Build history of the part. All positions in model axes, mm. A direction names the side the tool comes from. Round coordinates to 2 decimals unless told otherwise and drop trailing zeros. Loops run counter-clockwise (first coordinate to the right, second up) from the corner with the lowest first, then second, coordinate; pieces in that order, holes last. Notation, with made-up numbers: (-38.5, -8) - (-24.5, -8) arc R21 ccw to (-24.5, 24) - close; hole circle Ø7 at (2.25, 89). An arc over 180 degrees is marked (long way). Put each result on its own line as item: value. Start each with the question number.
from build123d import *

# Parameters (mm, degrees)
SKETCH_1_R               = 16.3
EXTRUDE_1_DEPTH          = 19.75
SKETCH_2_W               = 36.5
SKETCH_2_H               = 2.5
EXTRUDE_2_DEPTH          = 39.5
SKETCH_3_W               = 44.844436064
SKETCH_3_H               = 25.506740045
CUT_EXTRUDE_1_DEPTH      = 50
EXTRUDE_3_DEPTH          = 5.05
SKETCH_5_R               = 14.25
CUT_EXTRUDE_2_DEPTH      = 29.4
SKETCH_6_R               = 2.5
CUT_EXTRUDE_3_DEPTH      = 44.930797853
CUT_EXTRUDE_6_REACH      = 49.993
SKETCH_9_R               = 7.5
SKETCH_12_R              = 1.15
CUT_EXTRUDE_9_DEPTH      = 34.662664779
SKETCH_13_R              = 2
CUT_EXTRUDE_10_DEPTH     = 1
SKETCH_14_W              = 2.8
SKETCH_14_H              = 12
CUT_EXTRUDE_11_DEPTH     = 1.3
SKETCH_15_W              = 2.8
SKETCH_15_H              = 12
CUT_EXTRUDE_12_DEPTH     = 1.3
EXTRUDE_5_REACH          = 40.183
EXTRUDE_5_END_RADIUS     = 16.3
SKETCH_16_W              = 4
SKETCH_16_H              = 5
SKETCH_17_W              = 1
SKETCH_17_H              = 2
CUT_EXTRUDE_13_DEPTH     = 2.5
SKETCH_19_R              = 8.51898124
SKETCH_19_R_2            = 6.5
EXTRUDE_6_DEPTH          = 2.25
CUT_EXTRUDE_18_REACH     = 49.993
SKETCH_20_R              = 1.15
PATTERN_CIRCULAR_1_COUNT = 4
CUT_EXTRUDE_8_DEPTH      = 45.587021654
SKETCH_18_W              = 26.346157216
SKETCH_18_H              = 2.75
CUT_EXTRUDE_16_DEPTH     = 12.5
FILLET_1_R               = 2
FILLET_2_R               = 1
SKETCH_21_R              = 2.1
CUT_EXTRUDE_19_DEPTH     = 2.5
CUT_EXTRUDE_START        = -10
SKETCH_22_R              = 7.5
CUT_EXTRUDE_23_DEPTH     = 10
EXTRUDE_START            = -1
SKETCH_23_R              = 7.5
SKETCH_23_R_2            = 6.5
EXTRUDE_7_DEPTH          = 1
MOVE_FACE_3_BY           = 0.5


with BuildPart() as part:
    # 草图1 → 凸台-拉伸1 (new, symmetric)
    with BuildSketch(Plane(origin=(0, 0, 0), x_dir=(1, 0, 0), z_dir=(0, 1, 0))):
        with Locations(Location((0, 0, 0), (0, 0, 270))):
            Circle(SKETCH_1_R)
    extrude(amount=EXTRUDE_1_DEPTH, both=True)

    # 草图2 → 凸台-拉伸2 (add, through all)
    with BuildSketch(Plane.XZ.offset(19.75)):
        with Locations((3.6, -8.35)):
            Rectangle(SKETCH_2_W, SKETCH_2_H)
    extrude(amount=-EXTRUDE_2_DEPTH)

    # 草图3 → 切除-拉伸1 (cut)
    with BuildSketch(Plane.XZ.offset(19.75)):
        with Locations((-0.572218032, 5.653370022)):
            Rectangle(SKETCH_3_W, SKETCH_3_H)
    extrude(amount=-CUT_EXTRUDE_1_DEPTH, mode=Mode.SUBTRACT)

    # 草图4 → 凸台-拉伸3 (add)
    with BuildSketch(Plane.XZ.offset(19.75)):
        with BuildLine():
            Line((-14.65, -7.146152811), (-7.996542478, 4.549209646))
            ThreePointArc((-7.996542478, 4.549209646), (1.047927533, 9.140122969), (8.818653972, 2.621324497))
            ThreePointArc((8.818653972, 2.621324497), (13.721037439, -4.401937543), (21.85, -7.1))
            Line((21.85, -7.1), (-14.65, -7.146152811))
        make_face()
    extrude_3 = extrude(amount=-EXTRUDE_3_DEPTH)

    # 镜向1: 凸台-拉伸3 across plane
    add(extrude_3.mirror(Plane.ZX))

    # 草图5 → 切除-拉伸2 (cut)
    with BuildSketch(Plane(origin=(0, -14.7, 0), x_dir=(1, 0, 0), z_dir=(0, 1, 0))):
        Circle(SKETCH_5_R)
    extrude(amount=CUT_EXTRUDE_2_DEPTH, mode=Mode.SUBTRACT)

    # 草图6 → 切除-拉伸3 (cut, through all)
    with BuildSketch(Plane(origin=(0, -14.7, 0), x_dir=(1, 0, 0), z_dir=(0, 1, 0))):
        with Locations(Location((0, 0, 0), (0, 0, 270))):
            Circle(SKETCH_6_R)
    extrude(amount=-CUT_EXTRUDE_3_DEPTH, mode=Mode.SUBTRACT)

    # 草图9 → 切除-拉伸6 (cut, up to next)
    with BuildSketch(Plane(origin=(0, 19.75, 0), x_dir=(1, 0, 0), z_dir=(0, 1, 0)), mode=Mode.PRIVATE) as cut_extrude_6_sk1:
        with Locations(Location((0, 0, 0), (0, 0, 270))):
            Circle(SKETCH_9_R)
    cut_extrude_6_tool1 = extrude(cut_extrude_6_sk1.sketch, amount=-CUT_EXTRUDE_6_REACH, mode=Mode.PRIVATE) & part.part
    add(cut_extrude_6_tool1.solids().sort_by_distance((0, 19.75, 0))[0], mode=Mode.SUBTRACT)

    # 草图12 → 切除-拉伸9 (cut, through all)
    with BuildSketch(Plane.XY.offset(-7.1)):
        with Locations((17.5, 0)):
            Circle(SKETCH_12_R)
    extrude(amount=-CUT_EXTRUDE_9_DEPTH, mode=Mode.SUBTRACT)

    # 草图13 → 切除-拉伸10 (cut)
    with BuildSketch(Plane.XY.offset(-7.1)):
        with Locations((17.5, 0)):
            Circle(SKETCH_13_R)
    extrude(amount=-CUT_EXTRUDE_10_DEPTH, mode=Mode.SUBTRACT)

    # 草图14 → 切除-拉伸11 (cut)
    with BuildSketch(Plane.XY.offset(-7.1)):
        with Locations((21.85, 0)):
            Rectangle(SKETCH_14_W, SKETCH_14_H)
    extrude(amount=-CUT_EXTRUDE_11_DEPTH, mode=Mode.SUBTRACT)

    # 草图15 → 切除-拉伸12 (cut)
    with BuildSketch(Plane.XY.offset(-7.1)):
        with Locations((-14.672423113, 0)):
            Rectangle(SKETCH_15_W, SKETCH_15_H)
    extrude(amount=-CUT_EXTRUDE_12_DEPTH, mode=Mode.SUBTRACT)

    # 凸台-拉伸5: up to this cylinder (the profile starts outside it)
    extrude_5_end = Plane(origin=(0, 13.4, 0), z_dir=(0, -1, 0)) * Cylinder(EXTRUDE_5_END_RADIUS, 113.966, mode=Mode.PRIVATE)
    # 草图16 → 凸台-拉伸5 (add, up to the surface)
    with BuildSketch(Plane(origin=(0, 0, -15.1), x_dir=(-1, 0, 0), z_dir=(0, 0, -1)), mode=Mode.PRIVATE) as extrude_5_sk1:
        with Locations((11.65, 13.4)):
            Rectangle(SKETCH_16_W, SKETCH_16_H)
    extrude_5_tool1 = extrude(extrude_5_sk1.sketch, amount=-EXTRUDE_5_REACH, mode=Mode.PRIVATE) - extrude_5_end
    extrude_5 = extrude_5_tool1.solids().sort_by_distance((-11.65, 13.4, -15.1))[0]
    add(extrude_5)

    # 镜向4: 凸台-拉伸5 across plane
    add(extrude_5.mirror(Plane.ZX))

    # 草图17 → 切除-拉伸13 (cut)
    with BuildSketch(Plane(origin=(0, 0, -15.1), x_dir=(-1, 0, 0), z_dir=(0, 0, -1))):
        with Locations((11.65, 13.4)):
            Rectangle(SKETCH_17_W, SKETCH_17_H)
    cut_extrude_13 = extrude(amount=-CUT_EXTRUDE_13_DEPTH, mode=Mode.SUBTRACT)

    # 镜向5: 切除-拉伸13 across plane
    add(cut_extrude_13.mirror(Plane.ZX), mode=Mode.SUBTRACT)

    # 草图19 → 凸台-拉伸6 (add)
    with BuildSketch(Plane(origin=(0, 19.75, 0), x_dir=(1, 0, 0), z_dir=(0, 1, 0))):
        Circle(SKETCH_19_R)
        with Locations(Location((0, 0, 0), (0, 0, 270))):
            Circle(SKETCH_19_R_2, mode=Mode.SUBTRACT)
    extrude(amount=-EXTRUDE_6_DEPTH)

    # 草图20 → 切除-拉伸18 (cut, up to next)
    with BuildSketch(Plane.XZ.offset(19.75), mode=Mode.PRIVATE) as cut_extrude_18_sk1:
        with Locations(Location((0, 6, 0), (0, 0, 270))):
            Circle(SKETCH_20_R)
    cut_extrude_18_tool1 = extrude(cut_extrude_18_sk1.sketch, amount=-CUT_EXTRUDE_18_REACH, mode=Mode.PRIVATE) & part.part
    cut_extrude_18 = cut_extrude_18_tool1.solids().sort_by_distance((0, -19.75, 6))[0]
    add(cut_extrude_18, mode=Mode.SUBTRACT)

    # 阵列(圆周)1: 切除-拉伸18 ×4 about axis
    pattern_circular_1_axis = Axis((0, 0, 0), (0, 1, 0))
    for i in range(1, PATTERN_CIRCULAR_1_COUNT):
        add(cut_extrude_18.rotate(pattern_circular_1_axis, i * 360 / PATTERN_CIRCULAR_1_COUNT), mode=Mode.SUBTRACT)

    # 草图7 → 切除-拉伸8 (cut, through all)
    with BuildSketch(Plane.ZY.offset(14.65)):
        Polygon((-7.1, 19.75), (9.2, 18.323934785), (9.2, 19.75), align=None)
    cut_extrude_8 = extrude(amount=-CUT_EXTRUDE_8_DEPTH, mode=Mode.SUBTRACT)

    # 镜向3: 切除-拉伸8 across plane
    add(cut_extrude_8.mirror(Plane.ZX), mode=Mode.SUBTRACT)

    # 草图18 → 切除-拉伸16 (cut)
    with BuildSketch(Plane(origin=(0, 0, -9.6), x_dir=(-1, 0, 0), z_dir=(0, 0, -1))):
        with Locations((0, 18.375)):
            Rectangle(SKETCH_18_W, SKETCH_18_H)
    cut_extrude_16 = extrude(amount=CUT_EXTRUDE_16_DEPTH, mode=Mode.SUBTRACT)

    # 镜向6: 切除-拉伸16 across plane
    add(cut_extrude_16.mirror(Plane.ZX), mode=Mode.SUBTRACT)

    # 圆角1
    fillet_1_edges = [part.edges().sort_by_distance(p)[0] for p in [
        (12.355262037, 0, -7.1),
    ]]
    fillet(fillet_1_edges, radius=FILLET_1_R)

    # 圆角2
    fillet_2_edges = [part.edges().sort_by_distance(p)[0] for p in [
        (-12.355262037, 0, -7.1),
    ]]
    fillet(fillet_2_edges, radius=FILLET_2_R)

    # 草图21 → 切除-拉伸19 (cut)
    with BuildSketch(Plane.XZ.offset(19.75)):
        with Locations(Location((0, 6, 0), (0, 0, 270))):
            Circle(SKETCH_21_R)
        with Locations(Location((-6, 0, 0), (0, 0, 270))):
            Circle(SKETCH_21_R)
        with Locations(Location((6, 0, 0), (0, 0, 270))):
            Circle(SKETCH_21_R)
        with Locations(Location((0, -6, 0), (0, 0, 270))):
            Circle(SKETCH_21_R)
    extrude(amount=-CUT_EXTRUDE_19_DEPTH, mode=Mode.SUBTRACT)

    # 草图22 → 切除-拉伸23 (cut)
    with BuildSketch(Plane.XZ.offset(-17.5).offset(CUT_EXTRUDE_START)):
        with Locations(Location((0, 0, 0), (0, 0, 90))):
            Circle(SKETCH_22_R)
    extrude(amount=CUT_EXTRUDE_23_DEPTH, mode=Mode.SUBTRACT)

    # 草图23 → 凸台-拉伸7 (add)
    with BuildSketch(Plane.XZ.offset(-14.7).offset(EXTRUDE_START)):
        with Locations(Location((0, 0, 0), (0, 0, 288.796905035))):
            Circle(SKETCH_23_R)
        with Locations(Location((0, 0, 0), (0, 0, 270))):
            Circle(SKETCH_23_R_2, mode=Mode.SUBTRACT)
    extrude(amount=EXTRUDE_7_DEPTH)

    # Move Face 3: a face moved outward by 0.5
    extrude(part.faces().sort_by_distance((3.6131281, 14.7, -8.3875))[0], amount=MOVE_FACE_3_BY, dir=(0, -1, 0))


solid = part.part
1) Slice it at B-B, the plane z = 6. Write the cut outline in (x, y).
2) Which spindle directions (+Z, -Z, +X, -X, +Y, -Y) get a long thin tool onto all of the face, cutting with end or side? Do faces 1 (the face through (-7.15, -15.99, 0.05)), 2 (the face through (-12, 14.4, -14)), 3 (the face through (-3.955, 14.96, 5.158)). Say none if no direction does.
3) Slice it at A-A, the plane y = 15. Write the cut outline in (x, z), and give its area (3 significant figures).
4) Pull direction Z, two halves, no side cores. Call faces 4 (the face through (-12, 15.9, -13)), 5 (the face through (-1, -17.25, -7)), 6 (the face through (4.879, 19.674, -6.232)): pulls with the +Z half, pulls with the -Z half, needs draft (parallel to the pull), parting line crosses it, or undercut.
5) Drill centre lines: line 1 (Y direction, x = 4, z = -7.5); line 2 (Y direction, x = 4.5, z = -9.75); line 3 (Y direction, x = 7, z = -0.5). Where is each one in solid material? Low to high. Write a range as [from, to].
6) Slice it at D-D, the plane z = -13.75. Write the cut outline in (x, y), and give its area (3 significant figures).
7) Slice it at C-C, the plane x = 6. State how many separate pieces and enclosed holes the cut face has, and give its area (3 significant figures).
8) Drop flat-ended pins along their axis: pin 1 Ø1 at (y, z) = (-13, -14.5) entering from +X; pin 2 Ø5.5 at (y, z) = (13, -11.5) entering from -X; pin 3 Ø6 at (x, z) = (-5.5, -3.5) entering from +Y; pin 4 Ø2 at (x, y) = (17.5, 0) entering from +Z. Give the stop position or say it passes through.
Taken from the geometry:
1. outline: (-6.97, -18.6) - (-2.1, -18.6) - (-2.1, -17.25) - (-1.15, -17.25) - (-1.15, -14.7) - (-6.97, -14.7) - close; (-6.97, 14.2) - (-2.5, 14.2) - (-2.5, 15.7) - (-4.5, 15.7) - (-4.5, 18.6) - (-6.97, 18.6) - close; (1.15, -17.25) - (2.1, -17.25) - (2.1, -18.6) - (6.97, -18.6) - (6.97, -14.7) - (1.15, -14.7) - close; (2.5, 14.2) - (6.97, 14.2) - (6.97, 18.6) - (4.5, 18.6) - (4.5, 15.7) - (2.5, 15.7) - close
2. face 1: -Y
2. face 2: -Z
2. face 3: +Y
3. outline: (-14.67, -7.1) arc R16.3 ccw to (-14.65, -7.15) - (-14.65, -9.6) - (-13.65, -9.6) - (-13.65, -15.1) - (-9.65, -15.1) - (-9.65, -13.14) arc R16.3 ccw to (13.17, -9.6) - (21.85, -9.6) - (21.85, -7.1) arc R13.59 cw to (8.82, 2.62) arc R9.2 ccw to (-8, 4.55) - (-14.62, -7.1) - close; hole circle Ø13 at (0, 0)
3. area: 417 mm2
4. face 4: needs draft
4. face 5: undercut
4. face 6: pulls with the +Z half
5. line 1: y = [-19.75, -14.7], [14.2, 19.75]
5. line 2: y = [-17, -14.7], [14.2, 17]
5. line 3: y = [14.2, 15.7]
6. outline: (-13.65, -15.9) - (-9.65, -15.9) - (-9.65, -10.9) - (-13.65, -10.9) - close; (-13.65, 10.9) - (-9.65, 10.9) - (-9.65, 15.9) - (-13.65, 15.9) - close; (-8.75, -17) - (8.75, -17) - (8.75, 17) - (-8.75, 17) - close; hole (-12.15, -14.4) - (-11.15, -14.4) - (-11.15, -12.4) - (-12.15, -12.4) - close; hole (-12.15, 12.4) - (-11.15, 12.4) - (-11.15, 14.4) - (-12.15, 14.4) - close; hole (-3.74, -14.7) - (3.74, -14.7) - (3.74, 14.2) - (-3.74, 14.2) - close
6. area: 415 mm2
7. separate pieces: 3
7. enclosed holes: 0
7. area: 199 mm2
8. pin 1: stops at x = 8.35
8. pin 2: stops at x = -14.65
8. pin 3: stops at y = 19.7
8. pin 4: passes through
